Geometry check sheet. Reference: the model listing, model coordinates, mm. Face numbers are marked on the shaded views. A direction names the side the tool comes from. Coordinates: 2 decimals unless noted, no trailing zeros. Loops run counter-clockwise (first coordinate to the right, second up) from the corner with the lowest first, then second, coordinate; pieces in that order, holes last.
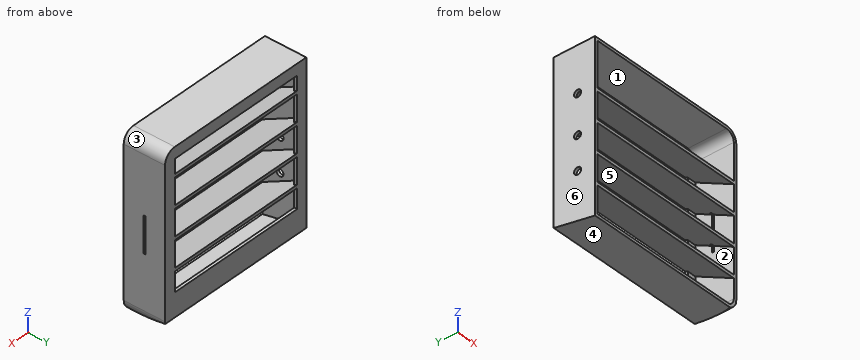
from build123d import *

# Parameters (mm, degrees)
F1_DEPTH    = 37
F2_T1_DEPTH = 342.8505669038
F3_T        = -2.54
F4_W        = 125.55387271
F4_H        = 111.9176980871
F5_DEPTH    = 25.4
F6_R        = 3.175
F7_DEPTH    = 19.05
F9_DEPTH    = 142.24
F10_W       = 2
F10_H       = 32
F11_DEPTH   = 5


# Not quite as in the source:
# - a fillet or chamfer that OpenCascade refuses, or shapes differently, is made with other operations: its cross-section is extruded or revolved along the edge and cut away or added


with BuildPart() as f1:
    # F0 (on Front) → F1 (new body)
    with BuildSketch(Plane.XZ):
        with BuildLine():
            Line((62.5, 75.5), (-72.5, 75.5))
            Line((-72.5, 75.5), (-72.5, -75.5))
            Line((-72.5, -75.5), (62.5, -75.5))
            ThreePointArc((62.5, -75.5), (69.5710678119, -72.5710678119), (72.5, -65.5))
            Line((72.5, -65.5), (72.5, 65.5))
            ThreePointArc((72.5, 65.5), (69.5710678119, 72.5710678119), (62.5, 75.5))
        make_face()
    extrude(amount=F1_DEPTH)

    # F2: chamfer of 40 x 8 on 1 edges, made by hand

    # F2_s2 → F2_t1 (cut)
    with BuildSketch(Plane.YZ.offset(-176.4252834519)):
        Polygon((-40, -75.5), (0, -67.5), (0, -75.5), align=None)
    extrude(amount=F2_T1_DEPTH, mode=Mode.SUBTRACT)

    # F3
    f3_openings = [f1.faces().sort_by_distance(p)[0] for p in [
        (-0.123954, -37, 0.284541),
    ]]
    offset(amount=F3_T, openings=f3_openings)

    # F4 (on face) → F5 (cut)
    with BuildSketch(Plane.XZ.offset(2.54)):
        with Locations((-0.276936355, 9.5411509565)):
            Rectangle(F4_W, F4_H)
    extrude(amount=-F5_DEPTH, mode=Mode.SUBTRACT)

    # F6 (on face) → F7 (cut)
    with BuildSketch(Plane(origin=(-72.5, 0, 0), x_dir=(0, -1, 0), z_dir=(-1, 0, 0))):
        with Locations((21.3561020792, 0)):
            Circle(F6_R)
        with Locations((21.3561020792, 35)):
            Circle(F6_R)
        with Locations((21.3561020792, -30)):
            Circle(F6_R)
    extrude(amount=-F7_DEPTH, mode=Mode.SUBTRACT)

    # F8 (on face) → F9 (join)
    with BuildSketch(Plane(origin=(69.96, 0, 0), x_dir=(0, -1, 0), z_dir=(-1, 0, 0))):
        Polygon((0, -28.8742875891), (37, -48.2893098931), (37, -45.4208615419), (0, -26.005839238), align=None)
        Polygon((0, -2.637839238), (37, -22.0528615419), (37, -19.1844131908), (0, 0.2306091132), align=None)
        Polygon((0, 23.5986091132), (37, 4.1835868092), (37, 7.0520351604), (0, 26.4670574643), align=None)
        Polygon((0, 49.8350574643), (37, 30.4200351604), (37, 33.2884835115), (0, 52.7035058155), align=None)
    extrude(amount=F9_DEPTH)

    # F10 (on face) → F11 (cut)
    with BuildSketch(Plane.YZ.offset(72.5)):
        with Locations((-18.3929149747, -1.5458973408)):
            Rectangle(F10_W, F10_H)
    extrude(amount=-F11_DEPTH, mode=Mode.SUBTRACT)


solid = f1.part
1) Section check C-C on y = -10. Record the cut outline in (x, z).
Data:
outline: (-72.5, -69.5) - (71.67, -69.5) arc R10 ccw to (72.5, -65.5) - (72.5, 65.5) arc R10 ccw to (62.5, 75.5) - (-72.5, 75.5) - close; hole (-69.96, -66.91) - (69.83, -66.91) arc R7.46 ccw to (69.96, -65.5) - (69.96, -34.12) - (-69.96, -34.12) - close; hole (-69.96, -31.25) - (69.96, -31.25) - (69.96, -7.89) - (-69.96, -7.89) - close; hole (-69.96, -5.02) - (69.96, -5.02) - (69.96, 18.35) - (-69.96, 18.35) - close; hole (-69.96, 21.22) - (69.96, 21.22) - (69.96, 44.59) - (-69.96, 44.59) - close; hole (-69.96, 47.46) - (69.96, 47.46) - (69.96, 65.5) arc R7.46 ccw to (62.5, 72.96) - (-69.96, 72.96) - close
2) Section check A-A on x = 20. Record the cut outline in (y, z).
Data:
outline: (-37, -74.9) - (0, -67.5) - (0, -46.42) - (-2.54, -46.42) - (-2.54, -65.42) - (-37, -72.31) - close; (-37, -48.29) - (0, -28.87) - (0, -26.01) - (-37, -45.42) - close; (-37, -22.05) - (0, -2.64) - (0, 0.23) - (-37, -19.18) - close; (-37, 4.18) - (0, 23.6) - (0, 26.47) - (-37, 7.05) - close; (-37, 30.42) - (0, 49.84) - (0, 52.7) - (-37, 33.29) - close; (-37, 72.96) - (-2.54, 72.96) - (-2.54, 65.5) - (0, 65.5) - (0, 75.5) - (-37, 75.5) - close
3) Access from +Z, -Z, +X, -X, +Y, -Y to the whole of each face (thin tool, end or side, straight path). Record for the marked faces 1, 2 and 3.
Data:
face 1: -Y
face 2: none
face 3: +Z, +X, +Y, -Y
4) Section check D-D on z = -35. Record the cut outline in (x, y).
Data:
outline: (-72.5, -37) - (-69.96, -37) - (-69.96, -17.14) - (69.96, -17.14) - (69.96, -37) - (72.5, -37) - (72.5, 0) - (62.5, 0) - (62.5, -2.54) - (69.96, -2.54) - (69.96, -11.67) - (-69.96, -11.67) - (-69.96, -2.54) - (-63.05, -2.54) - (-63.05, 0) - (-72.5, 0) - close
5) Depth check by flat-ended pin: pin 1 (6 mm diameter, centred on x = -46.5, y = -24.5, fed in from -Z); pin 2 (2 mm diameter, centred on x = 68, z = 10.5, fed in from -Y); pin 3 (2 mm diameter, centred on x = 70.5, y = -18.5, fed in from -Z). Enter the tip coordinate at first touch or a pass-through.
Data:
pin 1: stops at z = -73
pin 2: stops at y = -32.33
pin 3: stops at z = -71.4
6) Material ranges on probe 1 along X at (y, z) = (-3, -37.5); probe 2 along Z at (x, y) = (-13, -2.5); probe 3 along Z at (x, y) = (3, -10.5), recorded low to high.
Data:
probe 1: x = -72.5 to -69.96, 69.96 to 72.5
probe 2: z = -68 to -46.42, -30.19 to -27.32, -3.95 to -1.08, 22.29 to 25.16, 48.52 to 51.39, 65.5 to 75.5
probe 3: z = -69.6 to -67.01, -34.38 to -31.52, -8.15 to -5.28, 18.09 to 20.96, 44.33 to 47.19, 72.96 to 75.5
7) Section check B-B on z = 35. Record the cut outline in (x, y), and give its area (3 significant figures).
Data:
outline: (-72.5, -37) - (-69.96, -37) - (-69.96, -33.74) - (69.96, -33.74) - (69.96, -37) - (72.5, -37) - (72.5, 0) - (62.5, 0) - (62.5, -2.54) - (69.96, -2.54) - (69.96, -28.27) - (-69.96, -28.27) - (-69.96, -24.53) - (-72.5, -24.53) - close; (-72.5, -18.18) - (-69.96, -18.18) - (-69.96, -2.54) - (-63.05, -2.54) - (-63.05, 0) - (-72.5, 0) - close
area: 973 mm2
8) Mould release check, pull along Z, two halves, no side actions. Record for the marked faces 4, 5 and 6: +Z half, -Z half, draft (parallel to the pull), parting line (faces both ways), or undercut.
Data:
face 4: -Z half
face 5: undercut
face 6: draft
